Input: dimensioned drawing with shaded views. Units: mm. Origin: part minimum x, y, z. A direction names the side the tool comes from. Round coordinates to 2 decimals unless told otherwise and drop trailing zeros. Order: outer loops, then holes, each group sorted by start corner. A loop starts at its lowest first (then second) coordinate and runs counter-clockwise, first axis right, second up. Notation, with made-up numbers: M 77.25,-35.5 L 110.25,-35.5 A30 cw 110.25,-13.5 Z; hole C 4,-11.5 d4. An arc over 180 degrees is marked long. Put each result on its own line as item: value. Start each with the question number.
1) Draft query along Y for the marked faces 4, 5, 6 and 7. Return one class per face: pulls with the +Y half, pulls with the -Y half, needs draft (parallel to the pull), parting line crosses it, or undercut.
2) Section A-A, the plane y = 50. Return loops of the section in (x, z).
3) Section B-B, the plane z = 1.25. Return loops of the section in (x, y).
4) Section C-C, the plane x = 34. Return loops of the section in (y, z).
5) Material intervals for probe 1 along Y at (x, z) = (37.5, 2.25); probe 2 along X at (y, z) = (8, 1); probe 3 along Z at (x, y) = (36, 39), sorted ascending. Write a range as [from, to].
6) Access query for the marked faces 1, 2 and 3. Directions: +Z, -Z, +X, -X, +Y, -Y. A direction counts if a zero-diameter tool reaches every point of the face in a straight line with its end or side. Return the directions, or none.
7) Section D-D, the plane z = 7.5. Return loops of the section in (x, y).
8) First-contact query: P1, Ø2.5, axis at x = 2, z = 4, coming from the -Y side; P2, Ø5, axis at y = 60, z = 5, coming from the -X side; P3, Ø0.6, axis at x = 14, z = 1, coming from the +Y side. Flat tips, straight axial feed; report the tip coordinate or a pass-through.
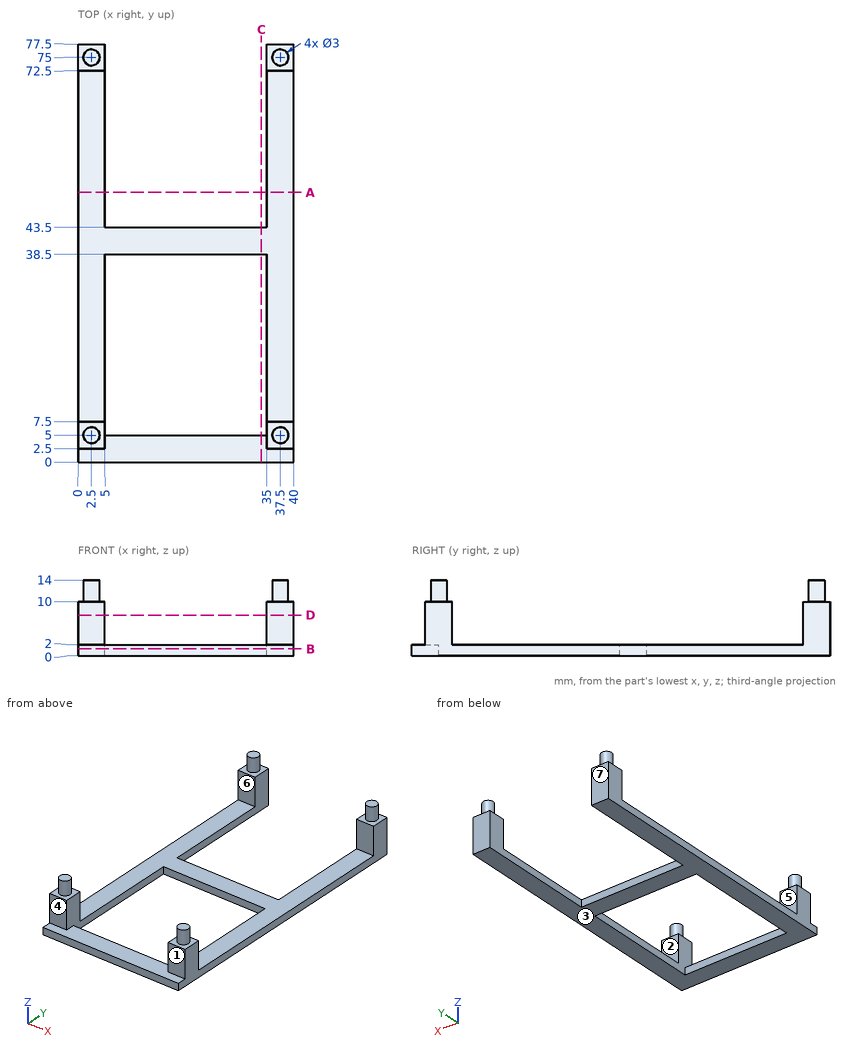
Result sheet:
1. face 4: pulls with the -Y half
1. face 5: undercut
1. face 6: undercut
1. face 7: pulls with the +Y half
2. outline: M 0,0 L 5,0 L 5,2 L 0,2 Z; M 35,0 L 40,0 L 40,2 L 35,2 Z
3. outline: M 0,0 L 40,0 L 40,77.5 L 35,77.5 L 35,43.5 L 5,43.5 L 5,77.5 L 0,77.5 Z; hole M 5,5 L 35,5 L 35,38.5 L 5,38.5 Z
4. outline: M 0,0 L 5,0 L 5,2 L 0,2 Z; M 38.5,0 L 43.5,0 L 43.5,2 L 38.5,2 Z
5. probe 1: y = [2.5, 7.5], [72.5, 77.5]
5. probe 2: x = [0, 5], [35, 40]
5. probe 3: z = [0, 2]
6. face 1: +Z, +X, -X, -Y
6. face 2: +Z, +X, -X
6. face 3: -Z, +X, -X, +Y, -Y
7. outline: M 0,2.5 L 5,2.5 L 5,7.5 L 0,7.5 Z; M 0,72.5 L 5,72.5 L 5,77.5 L 0,77.5 Z; M 35,2.5 L 40,2.5 L 40,7.5 L 35,7.5 Z; M 35,72.5 L 40,72.5 L 40,77.5 L 35,77.5 Z
8. P1: stops at y = 2.5
8. P2: passes through
8. P3: stops at y = 43.5
